Part model, mm, in its own coordinate system. Face numbers are marked on the shaded views. A direction names the side the tool comes from. Round coordinates to 2 decimals unless told otherwise and drop trailing zeros. Loops run counter-clockwise (first coordinate to the right, second up) from the corner with the lowest first, then second, coordinate; pieces in that order, holes last. Notation, with made-up numbers: (26, 79.25) - (52, 79.25) arc R25 cw to (52, 105.25) - close; hole circle Ø2 at (-28.75, 67). An arc over 180 degrees is marked (long way). Write each question's results on one line, items separated by ' | '. Start each with the question number.
(1) Mould opens along X. For the marked faces 1, 2, 3 and 4 say: released by +X, released by -X, zero draft, split by the parting line, or undercut.
(2) Cut at C-C, the plane y = 185. List the corners of the cut face in (x, z), then the cut area to 3 significant figures.
(3) Cut at B-B, the plane z = 80. List the corners of the cut face in (x, y).
(4) Flat gauge pins, fed straight in: P1, Ø16, axis at x = 40, z = -200, coming from the +Y side; P2, Ø1.5, axis at x = 158.5, y = 18, coming from the -Z side; P3, Ø2, axis at x = 109, y = 134, coming from the +Z side. Where does each tip first touch, or does it go through?
(5) Cut at D-D, the plane x = 53.5. List the corners of the cut face in (y, z), then the cut area to 3 significant figures.
(6) Cut at A-A, the plane x = 170. List the corners of the cut face in (y, z), then the cut area to 3 significant figures.
(7) Drill centre lines: L1, parallel to X at y = -0.5, z = 80; L2, parallel to Z at x = 170, y = -2; L3, parallel to Y at x = 128, z = 190.5. Where is each one in solid material? Low to high.
(8) Tool access for the marked faces 5, 6 and 7: list every direction of +Z, -Z, +X, -X, +Y, -Y with a clear straight run to the whole face (end or side of a thin tool).
Autodesk Inventor part; units mm, degrees
ref_plane "YZ Plane" through (0, 0, 0) normal (1, 0, 0) x (0, 1, 0)
ref_plane "XZ Plane" through (0, 0, 0) normal (0, 1, 0) x (-1, 0, 0)
ref_plane "XY Plane" through (0, 0, 0) normal (0, 0, 1) x (1, 0, 0)
sketch "Boceto1" plane through (0, 0, 0) normal (1, 0, 0) x (0, 1, 0)
  line L0 (10, 225) -> (-10, 225)
  line L1 (-10, 225) -> (-10, -225)
  line L2 (-10, -225) -> (10, -225)
  line L3 (10, -225) -> (10, 225)
  line L4 (10, 225) -> (-10, -225) construction
  line L5 (-10, 225) -> (10, -225) construction
  point P0 (0, 0)
  dimension "d0" = 20
  dimension "d1" = 450
extrude "Extrusión1" add sketch "Boceto1" along normal blind 210
sketch "Boceto2" plane through (0, 10, 225) normal (0, 1, 0) x (1, 0, 0)
  line L0 (0, 0) -> (0, 450)
  line L1 (210, 0) -> (210, 450)
  line L2 (0, 0) -> (210, 0)
  line L3 (210, 0) -> (210, 20)
  line L4 (210, 20) -> (0, 20)
  line L5 (0, 20) -> (0, 0)
  point P0 (0, 225)
  dimension "d4" = 20
extrude "Extrusión2" add sketch "Boceto2" along normal blind 80
sketch "Boceto3" plane through (0, 90, 225) normal (0, 1, 0) x (1, 0, 0)
  line L0 (0, 0) -> (210, 0)
  line L1 (0, 0) -> (210, 0)
  line L2 (210, 0) -> (210, -20)
  line L3 (210, -20) -> (0, -20)
  line L4 (0, -20) -> (0, 0)
  line L5 (0, 0) -> (210, 0)
  line L6 (210, 0) -> (210, 60)
  line L7 (210, 60) -> (0, 60)
  line L8 (0, 60) -> (0, 0)
  point P0 (0, 225)
  dimension "d7" = 20
  dimension "d8" = 210
  dimension "d9" = 60
extrude "Extrusión3" add sketch "Boceto3" along normal blind 130
sketch "Boceto4" plane through (0, 90, 245) normal (0, 0, 1) x (1, 0, 0)
  line L0 (10, 80) -> (200, 80)
  line L1 (200, 80) -> (200, 20)
  line L2 (200, 20) -> (10, 20)
  line L3 (10, 20) -> (10, 80)
  point P0 (0, -90)
  point P1 (0, 130)
  point P2 (210, 0)
  dimension "d12" = 190
  dimension "d13" = 60
extrude "Extrusión4" cut sketch "Boceto4" against normal blind 60
sketch "Boceto5" plane through (0, 220, 225) normal (0, 1, 0) x (1, 0, 0)
  line L0 (94.5, -1.5) -> (115.5, -1.5)
  line L1 (115.5, -1.5) -> (115.5, 41.5)
  line L2 (115.5, 41.5) -> (94.5, 41.5)
  line L3 (94.5, 41.5) -> (94.5, -1.5)
  line L4 (94.5, -1.5) -> (115.5, 41.5) construction
  line L5 (115.5, -1.5) -> (94.5, 41.5) construction
  point P0 (0, 225)
  point P1 (105, 20)
  dimension "d18" = 21
  dimension "d19" = 43
extrude "Extrusión5" cut sketch "Boceto5" against normal blind 43
sketch "Boceto6" plane through (0, 10, -225) normal (0, 1, 0) x (1, 0, 0)
  circle A0 centre (40, -305) radius 5
  circle A1 centre (40, -25) radius 5
  circle A2 centre (170, -305) radius 5
  circle A3 centre (170, -25) radius 5
  line L0 (0, -470) -> (210, -470)
  line L1 (0, 0) -> (210, 0)
  line L2 (0, 0) -> (0, -430)
  line L3 (210, 0) -> (210, -430)
  point P0 (0, -225)
  dimension "d23" = 10
  dimension "d24" = 10
  dimension "d25" = 10
  dimension "d26" = 10
  dimension "d27" = 165
  dimension "d28" = 25
  dimension "d29" = 25
  dimension "d30" = 165
  dimension "d31" = 40
  dimension "d32" = 40
  dimension "d33" = 40
  dimension "d34" = 40
extrude "Extrusión6" cut sketch "Boceto6" against normal blind 43
properties part number "base"
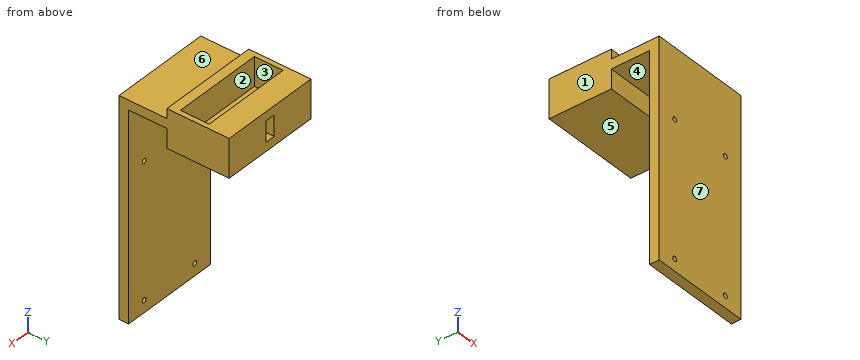
A:
1) face 1: released by -X | face 2: undercut | face 3: undercut | face 4: zero draft
2) outline: (0, 165) - (210, 165) - (210, 245) - (0, 245) - close; hole (94.5, 183.5) - (115.5, 183.5) - (115.5, 226.5) - (94.5, 226.5) - close | area: 15,900 mm2
3) outline: (0, -10) - (35, -10) - (35, 10) - (0, 10) - close; (45, -10) - (165, -10) - (165, 10) - (45, 10) - close; (175, -10) - (210, -10) - (210, 10) - (175, 10) - close
4) P1: y = 10 | P2: z = 205 | P3: z = 185
5) outline: (-10, -225) - (10, -225) - (10, 205) - (90, 205) - (90, 165) - (220, 165) - (220, 245) - (170, 245) - (170, 185) - (110, 185) - (110, 245) - (90, 245) - (90, 225) - (-10, 225) - close | area: 17,400 mm2
6) outline: (-10, -225) - (10, -225) - (10, -205) - (-10, -205) - close; (-10, -195) - (10, -195) - (10, 75) - (-10, 75) - close; (-10, 85) - (10, 85) - (10, 205) - (90, 205) - (90, 165) - (220, 165) - (220, 245) - (170, 245) - (170, 185) - (110, 185) - (110, 245) - (90, 245) - (90, 225) - (-10, 225) - close | area: 17,000 mm2
7) L1: 0 to 35, 45 to 165, 175 to 210 | L2: -225 to -205, -195 to 75, 85 to 225 | L3: -10 to 10, 90 to 110, 170 to 220
8) face 5: -Z, +X, -X, +Y | face 6: +Z, +X, -X, -Y | face 7: +Z, -Z, +X, -X, -Y
